from build123d import *

# Parameters (mm, degrees)
F0_R     = 10
F0_R_2   = 4.1
F1_DEPTH = 12
F2_R     = 1.6
F3_DEPTH = 25
F4_R     = 1.6
F5_DEPTH = 25
F6_R     = 6
F6_R_2   = 4.05
F7_DEPTH = 1.5
F8_SIZE  = 1


with BuildPart() as f1:
    # F0 (on Top) → F1 (new body)
    with BuildSketch(Plane.XY):
        Circle(F0_R)
        Circle(F0_R_2, mode=Mode.SUBTRACT)
    extrude(amount=F1_DEPTH)

    # F2 (on Front) → F3 (cut)
    with BuildSketch(Plane.XZ):
        with Locations((0, 6)):
            Circle(F2_R)
    extrude(amount=-F3_DEPTH, mode=Mode.SUBTRACT)

    # F4 (on Right) → F5 (cut)
    with BuildSketch(Plane.YZ):
        with Locations((0, 6)):
            Circle(F4_R)
    extrude(amount=-F5_DEPTH, mode=Mode.SUBTRACT)

    # F6 (on face) → F7 (join)
    with BuildSketch(Plane.XY.offset(12)):
        Circle(F6_R)
        Circle(F6_R_2, mode=Mode.SUBTRACT)
    extrude(amount=F7_DEPTH)

    # F8
    f8_edges = [f1.edges().sort_by_distance(p)[0] for p in [
        (-10, 0, 12),
    ]]
    chamfer(f8_edges, length=F8_SIZE)


solid = f1.part
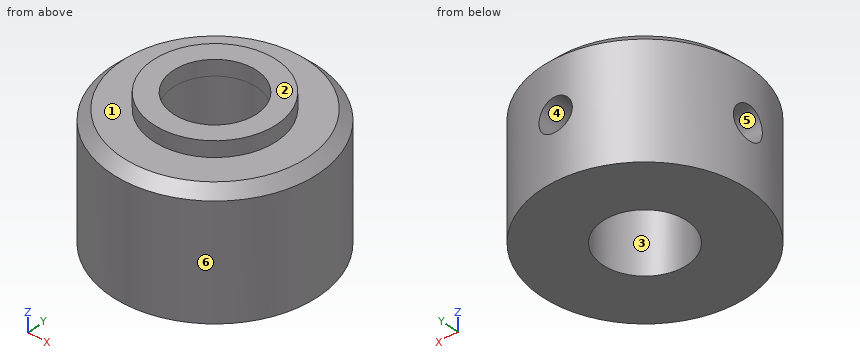
The listing builds one solid part. Answer for the finished solid, in the listing's coordinates (mm). Face numbers are marked on the shaded views. A direction names the side the tool comes from. Coordinates: 2 decimals unless noted, no trailing zeros. Write each loop counter-clockwise with the first axis right and the second up, starting at its lowest first coordinate (ties: lowest second). Pieces come first, ordered by that corner, then holes. Notation, with made-up numbers: M 65,-36.5 L 96,-36.5 A18 cw 96,-18.5 Z; hole C 49,71.5 d11. An arc over 180 degrees is marked long. Use one line per item in the form item = value.
Item 1: Find section B-B, the plane x = 0. Give the vertices of the cut face in (y, z).
Model answer:
outline = M -10,0 L -4.1,0 L -4.1,12 L -4.05,12 L -4.05,13.5 L -6,13.5 L -6,12 L -9,12 L -10,11 Z; M 4.05,12 L 4.1,12 L 4.1,7.6 L 10,7.6 L 10,11 L 9,12 L 6,12 L 6,13.5 L 4.05,13.5 Z; M 4.1,0 L 10,0 L 10,4.4 L 4.1,4.4 Z
Item 2: Find section C-C, the plane z = 5. Give the vertices of the cut face in (x, y), plus the area to 3 significant figures.
Model answer:
outline = M -9.92,-1.25 A10 ccw long 1.25,9.92 L 1.25,3.91 A4.1 cw long -3.91,-1.25 Z; M -9.92,1.25 L -3.91,1.25 A4.1 cw -1.25,3.91 L -1.25,9.92 A10 ccw Z
area = 232 mm2
Item 3: Find section D-D, the plane z = 12.75. Give the vertices of the cut face in (x, y), plus the area to 3 significant figures.
Model answer:
outline = C 0,0 d12; hole C 0,0 d8.1
area = 61.6 mm2
Item 4: The mould has two halves that part along X. Classify the marked faces 4, 5 and 6: released by +X, released by -X, zero draft, split by the parting line, or undercut.
Model answer:
face_4 = undercut
face_5 = zero draft
face_6 = split by the parting line
Item 5: Find the intervals of material crossed by probe 1 along Y at (x, z) = (0, 3.75); probe 2 along Y at (x, z) = (2, 7); probe 3 along X at (y, z) = (7, 6.75), in increasing order.
Model answer:
probe_1 = -10 to -4.1, 4.1 to 10
probe_2 = -9.8 to -3.58, 3.58 to 9.8
probe_3 = -7.14 to -1.41, 1.41 to 7.14
Item 6: Given P1, Ø3, axis at x = 0, y = 2.5, coming from the -Z side; P2, Ø6, axis at y = -4.5, z = 3, coming from the -X side; P3, Ø5, axis at x = -5.5, z = 3, coming from the +Y side; P4, Ø1.5, axis at x = 8, z = 9.5, coming from the -Y side, each flat-ended and moving along its own axis, determine where each tip first touches the part or whether it passes through.
Model answer:
P1 = through
P2 = -9.89
P3 = 9.54
P4 = -6.89
Item 7: For the marked faces 1, 2 and 3, determine the directions among +Z, -Z, +X, -X, +Y, -Y from which every point of the face is accessible in a straight line to the end or side of a thin tool.
Model answer:
face_1 = +Z
face_2 = +Z, +X, -X, +Y, -Y
face_3 = -Z
Item 8: Find section A-A, the plane y = 0. Give the vertices of the cut face in (x, z), plus the area to 3 significant figures.
Model answer:
outline = M -10,0 L -4.1,0 L -4.1,4.4 L -10,4.4 Z; M -10,7.6 L -4.1,7.6 L -4.1,12 L -4.05,12 L -4.05,13.5 L -6,13.5 L -6,12 L -9,12 L -10,11 Z; M 4.05,12 L 4.1,12 L 4.1,0 L 10,0 L 10,11 L 9,12 L 6,12 L 6,13.5 L 4.05,13.5 Z
area = 128 mm2
